Work out the finished part from the listing and answer in its coordinate system (mm). Face numbers are marked on the shaded views. A direction names the side the tool comes from. Coordinates: 2 decimals unless noted, no trailing zeros. Write each loop counter-clockwise with the first axis right and the second up, starting at its lowest first coordinate (ties: lowest second). Pieces come first, ordered by that corner, then holes. Notation, with made-up numbers: M -8.75,80.25 L 23.25,80.25 A17 cw 23.25,110.25 Z; hole C 68.25,13.5 d9. An arc over 180 degrees is marked long. Use CSV: the item, a comma, the result in double quotes.
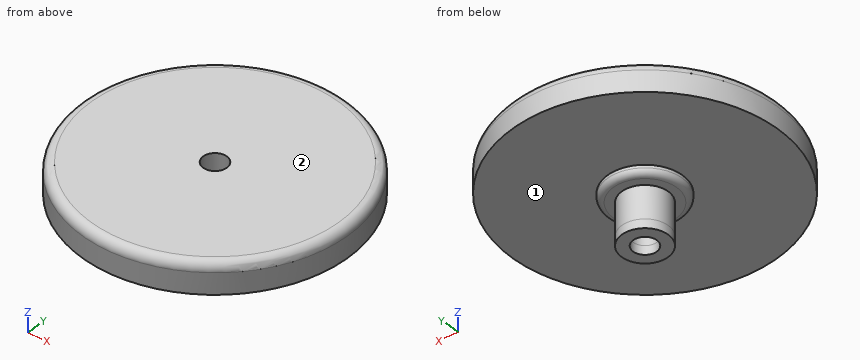
Autodesk Inventor part; units mm, degrees
ref_plane "YZ Plane" through (0, 0, 0) normal (1, 0, 0) x (0, 1, 0)
ref_plane "XZ Plane" through (0, 0, 0) normal (0, 1, 0) x (-1, 0, 0)
ref_plane "XY Plane" through (0, 0, 0) normal (0, 0, 1) x (1, 0, 0)
sketch "Sketch1" plane through (0, 0, 0) normal (0, 0, 1) x (1, 0, 0)
  circle A0 centre (0, 0) radius 3.925
  circle A1 centre (0, 0) radius 2
  dimension "d0" = 7.85
  dimension "d1" = 4
extrude "Extrusion1" add sketch "Sketch1" along normal blind 7
sketch "Sketch2" plane through (0, 0, 7) normal (0, 0, 1) x (1, 0, 0)
  circle A0 centre (0, 0) radius 22.5
  circle A1 centre (0, 0) radius 2
  dimension "d4" = 45
extrude "Extrusion2" add sketch "Sketch2" along normal blind 5.08
fillet "Fillet1" radius 1.5 1 edges at (-22.5, 0, 12.08)
sketch "Sketch4" plane through (0, 0, 7) normal (0, 0, -1) x (-1, 0, 0)
  circle A0 centre (0, 0) radius 3.925
  circle A1 centre (0, 0) radius 6.35
  dimension "d10" = 12.7
extrude "Extrusion4" add sketch "Sketch4" along normal blind 1.5
sketch "Sketch5" plane through (0, 0, 0) normal (0, 0, -1) x (-1, 0, 0)
  circle A0 centre (0, 0) radius 3.925
  circle A1 centre (0, 0) radius 2
fillet "Fillet2" radius 1 1 edges at (6.35, 0, 5.5)
extrude "Extrusion5" add sketch "Sketch5" along normal blind 1.5
properties part number "wheel_mrrover"
Item 1: A tool of negligible diameter and unlimited length cuts with its end or side. For the marked faces 1 and 2, from which of +Z, -Z, +X, -X, +Y, -Y can it reach the whole face along a straight path? Write none if from no direction.
Answer:
face 1,"-Z"
face 2,"+Z, +X, -X, +Y, -Y"
Item 2: The part is cut by section A-A (y = 0). Write down the section's boundary in (x, z) (3 decimals).
Answer:
outline,"M -22.5,7 L -6.35,7 L -6.35,6.5 A1 ccw -5.35,5.5 L -3.925,5.5 L -3.925,-1.5 L -2,-1.5 L -2,12.08 L -21,12.08 A1.5 ccw -22.5,10.58 Z; M 2,-1.5 L 3.925,-1.5 L 3.925,5.5 L 5.35,5.5 A1 ccw 6.35,6.5 L 6.35,7 L 22.5,7 L 22.5,10.58 A1.5 ccw 21,12.08 L 2,12.08 Z"
Item 3: The part is cut by section C-C (z = 3). Write down the section's boundary in (x, y) (3 decimals).
Answer:
outline,"C 0,0 d7.85; hole C 0,0 d4"
Item 4: Given pin 1 (2 mm diameter, centred on y = 5, z = 6.5, fed in from +X); pin 2 (3 mm diameter, centred on x = 0, y = 0, fed in from +Z); pin 3 (2 mm diameter, centred on x = -10.5, z = 7.5, fed in from +Y); pin 4 (12 mm diameter, centred on x = -12, y = 4, fed in from -Z), each flat-ended and moving along its own axis, determine where each tip first touches the part or whether it passes through.
Answer:
pin 1,"stops at x = 22.12"
pin 2,"passes through"
pin 3,"stops at y = 20.4"
pin 4,"stops at z = 7"
Item 5: Consider probe 1 along X at (y, z) = (0, 3.75) (3 decimals); probe 2 along Z at (x, y) = (-0.5, 18). Determine where each line is inside the solid, lowest interval first.
Answer:
probe 1,"x = -3.925 to -2, 2 to 3.925"
probe 2,"z = 7 to 12.08"
